Here's the drawing with two shaded views (mm, measured from the low corner). I have some questions. A direction names the side the tool comes from. Coordinates: 2 decimals unless noted, no trailing zeros. Write each loop counter-clockwise with the first axis right and the second up, starting at its lowest first coordinate (ties: lowest second). Pieces come first, ordered by that corner, then holes. Notation, with made-up numbers: (20.5, 19) -> (79.5, 19) arc R33 ccw to (79.5, 48) -> close; hole circle Ø5 at (82.25, 60.5). An arc over 180 degrees is marked (long way). Use a Markdown table: item, result. Add a question column.
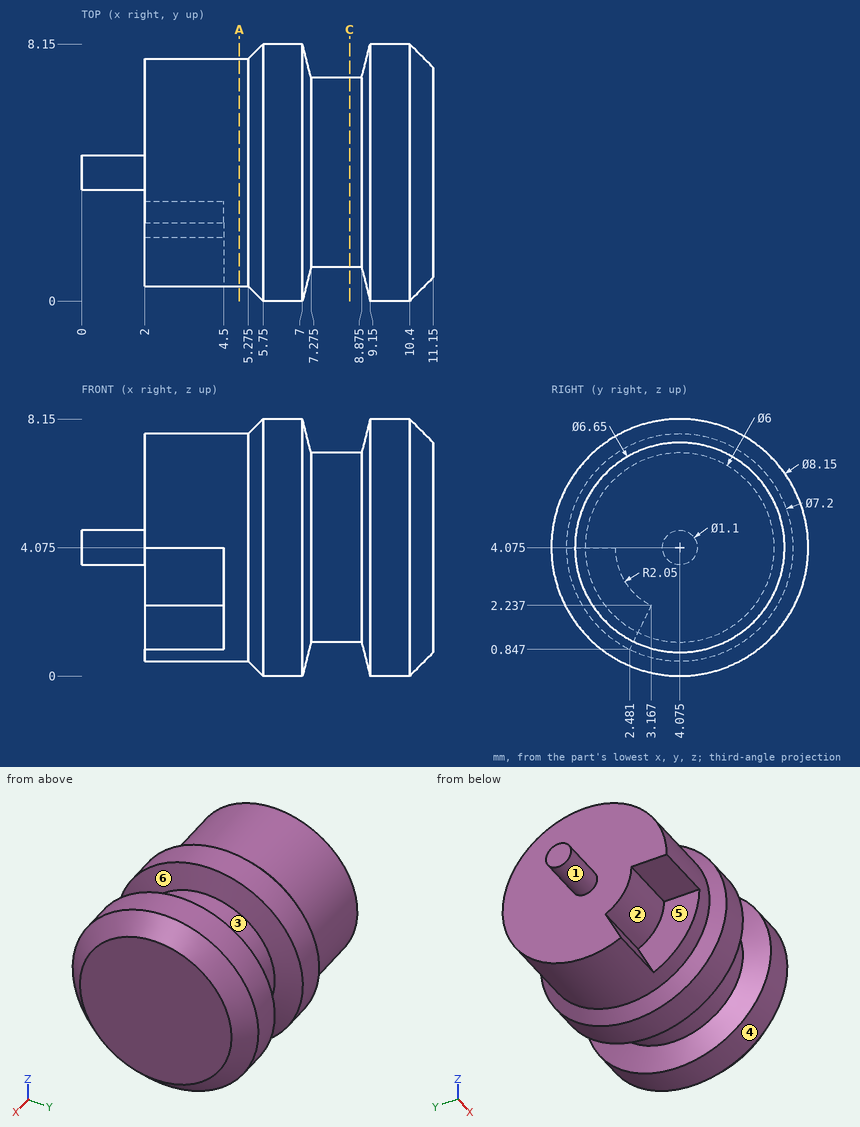
Q1. Will these pins go through, and if not, where does the flat tip stop? pin 1 (4 mm diameter, centred on x = 5, z = 6.5, fed in from +Y); pin 2 (1.2 mm diameter, centred on x = 3.5, y = 1, fed in from -Z) (3 decimals); pin 3 (1 mm diameter, centred on x = 10, y = 2.5, fed in from -Z) (1 decimal).
Q2. Suppose I cut it at C-C, the plane x = 8.5. Write out the boundary of the cut face in (y, z) (1 decimal).
Q3. Which directions (+Z, -Z, +X, -X, +Y, -Y) give clear straight access to the entire face, cutting with the end or side of a thin tool? Please do the marked faces 1, 2 and 3.
Q4. Suppose I cut it at A-A, the plane x = 5. Write out the boundary of the cut face in (y, z) (1 decimal).
Q5. Thinking about a two-plate mould opening in X: for the marked faces 4, 5 and 6, which applies, released by +X, released by -X, zero draft, split by the parting line, or undercut?
Q6. Please list where these lines run through material, in increasing order: line 1 (X direction, y = 2.5, z = 4.25); line 2 (X direction, y = 4.5, z = 7.25); line 3 (Y direction, x = 10, z = 4.25).
Answer key:
| question | item | result |
|---|---|---|
| 1 | pin 1 | stops at y = 8.11 |
| 1 | pin 2 | stops at z = 4.075 |
| 1 | pin 3 | stops at z = 0.1 |
| 2 | outline | circle Ø6 at (4.1, 4.1) |
| 3 | face 1 | -X |
| 3 | face 2 | -X, -Y |
| 3 | face 3 | none |
| 4 | outline | circle Ø7.2 at (4.1, 4.1) |
| 5 | face 4 | zero draft |
| 5 | face 5 | released by -X |
| 5 | face 6 | undercut |
| 6 | line 1 | x = 2 to 11.15 |
| 6 | line 2 | x = 2 to 7.22, 8.93 to 11.15 |
| 6 | line 3 | y = 0 to 8.15 |
